The model under review builds one solid part; all positions refer to its coordinate system, in mm. Face numbers are marked on the shaded views. A direction names the side the tool comes from. Give positions to 0.01 mm unless a question says otherwise; leave off trailing zeros. Order: outer loops, then holes, each group sorted by start corner. A loop starts at its lowest first (then second) coordinate and runs counter-clockwise, first axis right, second up. Notation, with made-up numbers: (-15, 6.5) -> (12, 6.5) arc R24 ccw to (12, 40.5) -> close; hole circle Ø7 at (19.5, 87). An arc over 180 degrees is marked (long way). Answer as a JSON object with one key per item and string values. Group by question number.
from build123d import *

# Parameters (mm, degrees)
F0_W      = 117.729
F0_H      = 81.661
F1_DEPTH  = 2.54
F2_W      = 117.729
F2_H      = 81.661
F3_DEPTH  = 2.032
F4_R      = 12.7
F5_W      = 17.78
F5_H      = 17.78
F6_DEPTH  = 4.572
F7_R      = 5.08
F13_R     = 3.048
F14_DEPTH = 4.573


# Not quite as in the source:
# - a feature of the source that left no trace in its solid (it failed there, or was rolled back) is left out
# - a pattern or mirror of a feature is missing from the dataset's text; its kind, count and spacing are read off the source's solid


with BuildPart() as f1:
    # F0 (on Top) → F1 (new body)
    with BuildSketch(Plane.XY):
        with Locations((-58.8645, 40.8305)):
            Rectangle(F0_W, F0_H)
    extrude(amount=F1_DEPTH)

    # F2 (on face) → F3 (join)
    with BuildSketch(Plane.XY.offset(2.54)):
        with Locations((-58.8645, 40.8305)):
            Rectangle(F2_W, F2_H)
        with BuildLine():
            ThreePointArc((-5.08, 14.605), (-7.8698079092, 7.8698079092), (-14.605, 5.08))
            Line((-14.605, 5.08), (-103.124, 5.08))
            ThreePointArc((-103.124, 5.08), (-109.8591920908, 7.8698079092), (-112.649, 14.605))
            Line((-112.649, 14.605), (-112.649, 32.2905))
            ThreePointArc((-112.649, 32.2905), (-111.9050512242, 34.0865512242), (-110.109, 34.8305))
            Line((-110.109, 34.8305), (-108.3945, 34.8305))
            ThreePointArc((-108.3945, 34.8305), (-105.6939926316, 35.4725843649), (-103.5714697827, 37.2614133489))
            ThreePointArc((-103.5714697827, 37.2614133489), (-102.67293511, 38.0186842855), (-101.529720324, 38.2905))
            Line((-101.529720324, 38.2905), (-58.8645, 38.2905))
            Line((-58.8645, 38.2905), (-16.199279676, 38.2905))
            ThreePointArc((-16.199279676, 38.2905), (-15.05606489, 38.0186842855), (-14.1575302173, 37.2614133489))
            ThreePointArc((-14.1575302173, 37.2614133489), (-12.0350073684, 35.4725843649), (-9.3345, 34.8305))
            Line((-9.3345, 34.8305), (-7.62, 34.8305))
            ThreePointArc((-7.62, 34.8305), (-5.8239487758, 34.0865512242), (-5.08, 32.2905))
            Line((-5.08, 32.2905), (-5.08, 14.605))
        make_face(mode=Mode.SUBTRACT)
        with BuildLine():
            Line((-103.124, 76.581), (-14.605, 76.581))
            ThreePointArc((-14.605, 76.581), (-7.8698079092, 73.7911920908), (-5.08, 67.056))
            Line((-5.08, 67.056), (-5.08, 49.3705))
            ThreePointArc((-5.08, 49.3705), (-5.8239487758, 47.5744487758), (-7.62, 46.8305))
            Line((-7.62, 46.8305), (-9.3345, 46.8305))
            ThreePointArc((-9.3345, 46.8305), (-12.0350073684, 46.1884156351), (-14.1575302173, 44.3995866511))
            ThreePointArc((-14.1575302173, 44.3995866511), (-15.05606489, 43.6423157145), (-16.199279676, 43.3705))
            Line((-16.199279676, 43.3705), (-58.8645, 43.3705))
            Line((-58.8645, 43.3705), (-101.529720324, 43.3705))
            ThreePointArc((-101.529720324, 43.3705), (-102.67293511, 43.6423157145), (-103.5714697827, 44.3995866511))
            ThreePointArc((-103.5714697827, 44.3995866511), (-105.6939926316, 46.1884156351), (-108.3945, 46.8305))
            Line((-108.3945, 46.8305), (-110.109, 46.8305))
            ThreePointArc((-110.109, 46.8305), (-111.9050512242, 47.5744487758), (-112.649, 49.3705))
            Line((-112.649, 49.3705), (-112.649, 67.056))
            ThreePointArc((-112.649, 67.056), (-109.8591920908, 73.7911920908), (-103.124, 76.581))
        make_face(mode=Mode.SUBTRACT)
    extrude(amount=F3_DEPTH)

    # F4
    f4_edges = [f1.edges().sort_by_distance(p)[0] for p in [
        (-117.729, 0, 2.286),
        (-117.729, 81.661, 2.286),
        (0, 81.661, 2.286),
        (0, 0, 2.286),
    ]]
    fillet(f4_edges, radius=F4_R)

    # F5 (on face) → F6 (join, through all)
    with BuildSketch(Plane.XY.offset(4.572)):
        with Locations((8.89, 40.8305)):
            Rectangle(F5_W, F5_H)
    f6 = extrude(amount=-F6_DEPTH)

    # F6_copies: F6 across plane
    add(f6.mirror(Plane(origin=(-58.8645, 0, 0), x_dir=(0, 0, -1), z_dir=(-1, 0, 0))))

    # F7
    f7_edges = [f1.edges().sort_by_distance(p)[0] for p in [
        (0, 31.9405, 2.286),
        (0, 49.7205, 2.286),
        (17.78, 49.7205, 2.286),
        (17.78, 31.9405, 2.286),
        (-117.729, 49.7205, 2.286),
        (-117.729, 31.9405, 2.286),
        (-135.509, 49.7205, 2.286),
        (-135.509, 31.9405, 2.286),
    ]]
    fillet(f7_edges, radius=F7_R)

    # F13 (on face) → F14 (cut, through all)
    with BuildSketch(Plane.XY.offset(4.572)):
        with Locations((9.398, 40.8305)):
            Circle(F13_R)
        with Locations((-127.127, 40.8305)):
            Circle(F13_R)
    extrude(amount=-F14_DEPTH, mode=Mode.SUBTRACT)


solid = f1.part
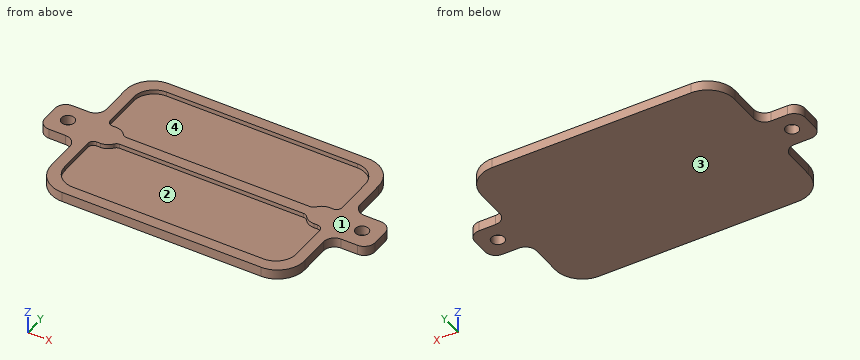
1. Take a section at D-D on y = 7. Give the boundary of the cut face in (x, z), plus the area to 3 significant figures.
2. Machinability: for the marked faces 1 and 2, which of the approach directions +Z, -Z, +X, -X, +Y, -Y give a long, thin tool a straight path to every point of the face, cutting with its end or side? Answer none if there is none.
3. Take a section at B-B on x = -50. Give the boundary of the cut face in (y, z).
4. For probe 1 along Y at (x, z) = (-34, 3.7); probe 2 along Y at (x, z) = (-11, 4.35); probe 3 along Z at (x, y) = (-49, 35.5), list the stretches that pass through material, from the lowest coordinate up. Write a range as [from, to].
5. For pin 1 (2.5 mm diameter, centred on x = 10.5, z = 3, fed in from +Y); pin 2 (0.5 mm diameter, centred on x = -8.5, z = 3.5, fed in from -Y); pin 3 (4 mm diameter, centred on x = -76, y = 15.5, fed in from +Z), all flat-tipped, find the tip position at first contact; note any pin that passes through.
6. Take a section at C-C on y = 18. Give the boundary of the cut face in (x, z), plus the area to 3 significant figures.
7. Take a section at A-A on z = 1.4. Give the boundary of the cut face in (x, y), plus the area to 3 significant figures.
8. Draft analysis for pull direction X (two halves, no side actions). For the marked faces 3 and 4, state which applies: pulls with the +X half, pulls with the -X half, needs draft (parallel to the pull), parting line crosses it, or undercut.
Checks:
{
 "1": {"outline": "(-116.38, 0) -> (-1.35, 0) -> (-1.35, 4.57) -> (-8.87, 4.57) -> (-8.87, 2.54) -> (-108.86, 2.54) -> (-108.86, 4.57) -> (-116.38, 4.57) -> close", "area": "323 mm2"},
 "2": {"face 1": "+Z, +X, -X, +Y, -Y", "face 2": "+Z"},
 "3": {"outline": "(0, 0) -> (81.66, 0) -> (81.66, 4.57) -> (76.58, 4.57) -> (76.58, 2.54) -> (43.37, 2.54) -> (43.37, 4.57) -> (38.29, 4.57) -> (38.29, 2.54) -> (5.08, 2.54) -> (5.08, 4.57) -> (0, 4.57) -> close"},
 "4": {"probe 1": "y = [0, 5.08], [38.29, 43.37], [76.58, 81.66]", "probe 2": "y = [0.11, 5.79], [35.07, 46.59], [75.87, 81.55]", "probe 3": "z = [0, 2.54]"},
 "5": {"pin 1": "stops at y = 49.72", "pin 2": "stops at y = 0.63", "pin 3": "stops at z = 2.54"},
 "6": {"outline": "(-117.73, 0) -> (0, 0) -> (0, 4.57) -> (-5.08, 4.57) -> (-5.08, 2.54) -> (-112.65, 2.54) -> (-112.65, 4.57) -> (-117.73, 4.57) -> close", "area": "320 mm2"},
 "7": {"outline": "(-135.51, 37.02) arc R5.08 ccw to (-130.43, 31.94) -> (-122.81, 31.94) arc R5.08 cw to (-117.73, 26.86) -> (-117.73, 12.7) arc R12.7 ccw to (-105.03, 0) -> (-12.7, 0) arc R12.7 ccw to (0, 12.7) -> (0, 26.86) arc R5.08 cw to (5.08, 31.94) -> (12.7, 31.94) arc R5.08 ccw to (17.78, 37.02) -> (17.78, 44.64) arc R5.08 ccw to (12.7, 49.72) -> (5.08, 49.72) arc R5.08 cw to (0, 54.8) -> (0, 68.96) arc R12.7 ccw to (-12.7, 81.66) -> (-105.03, 81.66) arc R12.7 ccw to (-117.73, 68.96) -> (-117.73, 54.8) arc R5.08 cw to (-122.81, 49.72) -> (-130.43, 49.72) arc R5.08 ccw to (-135.51, 44.64) -> close; hole circle Ø6.1 at (-127.13, 40.83); hole circle Ø6.1 at (9.4, 40.83)", "area": "10,000 mm2"},
 "8": {"face 3": "needs draft", "face 4": "undercut"}
}
